Study the drawing (mm; zero at the part's minimum x, y, z) and answer. Give positions to 0.01 mm unless a question says otherwise; leave off trailing zeros. Order: outer loops, then holes, each group sorted by start corner. A loop starts at its lowest first (then second) coordinate and runs counter-clockwise, first axis right, second up. Notation, with made-up numbers: (5, 2.25) - (36, 2.25) arc R30 cw to (36, 28.25) - close; hole circle Ø9 at (-37, 17). An arc over 180 degrees is marked (long way). Return JSON: item names as keys, results as strings.
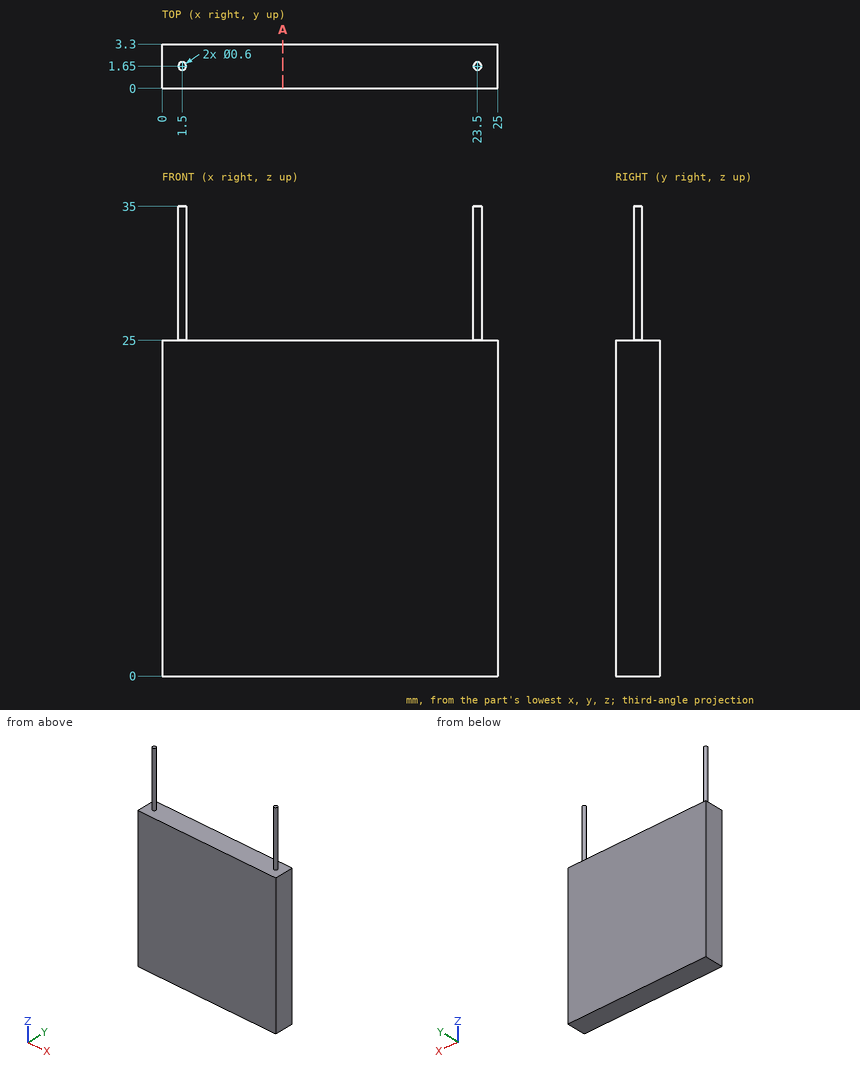
Q1. Given pin 1 (1.5 mm diameter, centred on x = 21.5, y = 0.5, fed in from +Z), flat-ended and moving along its own axis, determine where the tip first touches the part or whether it passes through.
Values:
{"pin 1": "stops at z = 25"}
Q2. Consider L1, parallel to Z at x = 3, y = 0.9; L2, parallel to X at y = 1.9, z = 31. Determine where each line is inside the solid, lowest interval first.
Values:
{"L1": "z = 0 to 25", "L2": "x = 1.33 to 1.67, 23.33 to 23.67"}
Q3. A cutting plane is placed at A-A (x = 9). Write down the section's boundary in (y, z), and give its area (3 significant figures).
Values:
{"outline": "(0, 0) - (3.3, 0) - (3.3, 25) - (0, 25) - close", "area": "82.5 mm²"}
